Read the model definition and answer for the solid it produces. Units are mm, in the model's axes. A direction names the side the tool comes from. Give positions to 0.01 mm unless a question says otherwise; leave off trailing zeros. Order: outer loops, then holes, each group sorted by start corner. A loop starts at its lowest first (then second) coordinate and runs counter-clockwise, first axis right, second up. Notation, with made-up numbers: (-2, 89) - (41, 89) arc R8 ccw to (41, 102) - close; hole circle Ø6 at (62.5, 12.5). An arc over 180 degrees is marked (long way). Use a Markdown table: item, result. Add a question column.
1. Consider L1, parallel to Y at x = 105, z = 12.25; L2, parallel to Y at x = 47, z = 12.75; L3, parallel to Y at x = 18.5, z = 13.5. Determine where each line is inside the solid, lowest interval first.
2. Which of the six approach directions +Z, -Z, +X, -X, +Y, -Y give full straight-line access (tool end or side, diameter ignored) to faces 4 (the cylindrical face through (10, 24, 18)), 5 (the cylindrical face through (26.36, 10.53, 7.4)), 6 (the cylindrical face through (93.35, 23.77, 7.4)), 7 (the flat face through (-44.96, 12.64, 7.4)), 8 (the cylindrical face through (116.804, -24.289, 7.395))?
3. A cutting plane is placed at A-A on x = 105. Determine the outline of the cut face in (y, z).
4. For a pull along X with two mould halves and no side action, classify faces 1 (the flat face through (-44.78, -12.52, 7.4)), 2 (the cylindrical face through (28.44, -10.8, 7.4)), 3 (the flat face through (-24, 26, 7)) as released by +X, released by -X, zero draft, split by the parting line, or undercut.
5. A cutting plane is placed at B-B on y = 63. Determine the outline of the cut face in (x, z).
6. A cutting plane is placed at C-C on z = 22.5. State how many separate pieces and enclosed holes the cut face has, and give its area (3 significant figures).
7. Flat-ended cylindrical pins translate along their axes: P1, Ø5, axis at y = 64.5, z = 8, coming from the -X side; P2, Ø4, axis at x = 37.5, z = 8.5, coming from the +Y side; P3, Ø8, axis at x = 105, y = 37, coming from the -Z side; P4, Ø12, axis at x = 74, z = 11, coming from the +Y side. Find the tip coordinate at first contact, or state that the pin passes through.
8. A cutting plane is placed at D-D on x = -41. Determine the outline of the cut face in (y, z).
```python
from build123d import *

# Parameters (mm, degrees)
EXTRUDE_1_DEPTH = 15
SKETCH_1_3_R    = 39
SKETCH_1_3_R_2  = 5
SKETCH_1_3_R_3  = 12.5
SKETCH_1_3_R_4  = 26
SKETCH_1_3_R_5  = 4
SKETCH_1_3_R_6  = 7.5
EXTRUDE_4_DEPTH = 25
EXTRUDE_START   = -10
EXTRUDE_5_DEPTH = 10


with BuildPart() as part:
    # Sketch 1 → Extrude 1 (new body)
    with BuildSketch(Plane.XY):
        with BuildLine():
            Line((0, 26), (-48.486121811, 26))
            ThreePointArc((-48.486121811, 26), (-53.271581944, 22.448920743), (-51.259622792, 16.839748528))
            Line((-51.259622792, 16.839748528), (-38.480754415, 8.320502943))
            ThreePointArc((-38.480754415, 8.320502943), (-34.027756377, 0), (-38.480754415, -8.320502943))
            Line((-38.480754415, -8.320502943), (-51.259622792, -16.839748528))
            ThreePointArc((-51.259622792, -16.839748528), (-53.271581944, -22.448920743), (-48.486121811, -26))
            Line((-48.486121811, -26), (-18, -26))
            ThreePointArc((-18, -26), (-5.272077939, -31.272077939), (0, -44))
            Line((0, -44), (145, -44))
            ThreePointArc((145, -44), (139.727922061, -31.272077939), (127, -26))
            Line((127, -26), (121, -26))
            ThreePointArc((121, -26), (116.757359313, -24.242640687), (115, -20))
            Line((115, -20), (115, 18.267461507))
            ThreePointArc((115, 18.267461507), (116.609042768, 23.70729944), (120.918367347, 27.396550996))
            ThreePointArc((120.918367347, 27.396550996), (105, 24), (89.081632653, 27.396550996))
            ThreePointArc((89.081632653, 27.396550996), (93.390957232, 23.70729944), (95, 18.267461507))
            Line((95, 18.267461507), (95, 15))
            ThreePointArc((95, 15), (93.242640687, 10.757359313), (89, 9))
            Line((89, 9), (32.726136344, 9))
            ThreePointArc((32.726136344, 9), (26.272455224, 10.576232455), (21.271988624, 14.95))
            ThreePointArc((21.271988624, 14.95), (24.789833644, 7.839907391), (26, 0))
            ThreePointArc((26, 0), (-18.384776311, -18.384776311), (0, 26))
        make_face()
        with BuildLine():
            Line((89, -23), (32.726136344, -23))
            ThreePointArc((32.726136344, -23), (28.483495657, -21.242640687), (26.726136344, -17))
            Line((26.726136344, -17), (26.726136344, -15))
            ThreePointArc((26.726136344, -15), (28.483495657, -10.757359313), (32.726136344, -9))
            Line((32.726136344, -9), (89, -9))
            ThreePointArc((89, -9), (93.242640687, -10.757359313), (95, -15))
            Line((95, -15), (95, -17))
            ThreePointArc((95, -17), (93.242640687, -21.242640687), (89, -23))
        make_face(mode=Mode.SUBTRACT)
    extrude(amount=EXTRUDE_1_DEPTH)

    # Sketch 1_3 → Extrude 4 (add)
    # profile 1 of 2: a face of its own
    with BuildSketch(Plane.XY):
        with Locations(Location((105, 63, 0), (0, 0, 245.910493888))):
            Circle(SKETCH_1_3_R)
        with Locations((129.727469424, 54.965558146)):
            Circle(SKETCH_1_3_R_2, mode=Mode.SUBTRACT)
        with Locations((120.28241656, 84.034441854)):
            Circle(SKETCH_1_3_R_2, mode=Mode.SUBTRACT)
        with Locations((89.71758344, 84.034441854)):
            Circle(SKETCH_1_3_R_2, mode=Mode.SUBTRACT)
        with Locations((80.272530576, 54.965558146)):
            Circle(SKETCH_1_3_R_2, mode=Mode.SUBTRACT)
        with Locations((105, 37)):
            Circle(SKETCH_1_3_R_2, mode=Mode.SUBTRACT)
        with Locations((105, 63)):
            Circle(SKETCH_1_3_R_3, mode=Mode.SUBTRACT)
    # profile 2 of 2: a face of its own
    with BuildSketch(Plane.XY):
        with Locations(Location((0, 0, 0), (0, 0, 90))):
            Circle(SKETCH_1_3_R_4)
        with Locations((-9, 15.588457268)):
            Circle(SKETCH_1_3_R_5, mode=Mode.SUBTRACT)
        with Locations((-9, -15.588457268)):
            Circle(SKETCH_1_3_R_5, mode=Mode.SUBTRACT)
        with Locations((18, 0)):
            Circle(SKETCH_1_3_R_5, mode=Mode.SUBTRACT)
        Circle(SKETCH_1_3_R_6, mode=Mode.SUBTRACT)
    extrude(amount=EXTRUDE_4_DEPTH)

    # Sketch 1_4 → Extrude 5 (add)
    with BuildSketch(Plane.XY.offset(EXTRUDE_START)):
        with BuildLine():
            Line((32.726136344, -23), (89, -23))
            ThreePointArc((89, -23), (93.242640687, -21.242640687), (95, -17))
            Line((95, -17), (95, -15))
            ThreePointArc((95, -15), (93.242640687, -10.757359313), (89, -9))
            Line((89, -9), (32.726136344, -9))
            ThreePointArc((32.726136344, -9), (28.483495657, -10.757359313), (26.726136344, -15))
            Line((26.726136344, -15), (26.726136344, -17))
            ThreePointArc((26.726136344, -17), (28.483495657, -21.242640687), (32.726136344, -23))
        make_face()
    extrude(amount=EXTRUDE_5_DEPTH)


with BuildPart() as extrude_5_kept_piece:
    # of the separate pieces the step leaves, the one the design keeps (extrude_5_pieces_kept)
    add(part.part.solids().sort_by_distance((0, 26, 0))[0])


solid = extrude_5_kept_piece.part
```
Output values:
| question | item | result |
|---|---|---|
| 1 | L1 | -44 to 32, 42 to 50.5, 75.5 to 102 |
| 1 | L2 | -44 to -23, -9 to 9 |
| 1 | L3 | -44 to -3.97, 3.97 to 18.27 |
| 2 | face 4 | +Z |
| 2 | face 5 | +Z, -Z, +Y |
| 2 | face 6 | +Z, -Z |
| 2 | face 7 | +Z, -Z, -X |
| 2 | face 8 | +Z, -Z, +X |
| 3 | outline | (-44, 0) - (32, 0) - (32, 25) - (24, 25) - (24, 15) - (-44, 15) - close; (42, 0) - (50.5, 0) - (50.5, 25) - (42, 25) - close; (75.5, 0) - (102, 0) - (102, 25) - (75.5, 25) - close |
| 4 | face 1 | released by -X |
| 4 | face 2 | undercut |
| 4 | face 3 | zero draft |
| 5 | outline | (66, 0) - (92.5, 0) - (92.5, 25) - (66, 25) - close; (117.5, 0) - (144, 0) - (144, 25) - (117.5, 25) - close |
| 6 | separate pieces | 2 |
| 6 | enclosed holes | 10 |
| 6 | area | 5,690 mm² |
| 7 | P1 | x = 66 |
| 7 | P2 | y = 9 |
| 7 | P3 | through |
| 7 | P4 | y = 92.93 |
| 8 | outline | (-26, 0) - (-10, 0) - (-10, 15) - (-26, 15) - close; (10, 0) - (26, 0) - (26, 15) - (10, 15) - close |
